```python
from build123d import *

# Parameters (mm, degrees)
F3_R     = 1.905
F7_W     = 78.89875
F7_H     = 0.5301288674
F8_DEPTH = 171.451


with BuildPart() as f1:
    # F0 (on Top) → F1 (revolve)
    with BuildSketch(Plane.XY):
        Polygon((-46.0375, 0), (-160.3375, 0), (-160.3375, -6.35), (-109.5375, -6.35), (-109.5375, -4.7625), (-84.1375, -4.7625), (-84.1375, -1.905), (84.1375, -1.905), (84.1375, -2.38125), (109.5375, -2.38125), (109.5375, -6.35), (134.9375, -6.35), (134.9375, -3.175), (160.3375, -3.175), (160.3375, 0), align=None)
    revolve(axis=Axis((40.7620462889, 0, 0), (1, 0, 0)))

    # F4: sweep along a path in F0
    with BuildLine(Plane.XY) as f4_path:
        Line((171.45, 73.81875), (45.1552021657, 73.81875))
        ThreePointArc((45.1552021657, 73.81875), (42.9987538677, 73.4413734385), (41.0986183394, 72.3540982639))
        Line((41.0986183394, 72.3540982639), (-46.0375, 0))
    # F3 (on plane+point) → F4 (sweep)
    with BuildSketch(Plane.YZ.offset(171.45)):
        with Locations((73.81875, 0)):
            Circle(F3_R)
    sweep(path=f4_path.line)

    # F5 (on Top) → F6 (revolve)
    with BuildSketch(Plane.XY):
        Polygon((95.25, 73.81875), (171.45, 73.81875), (171.45, 76.99375), (146.05, 76.99375), (146.05, 80.16875), (120.65, 80.16875), (120.65, 78.58125), (95.25, 78.58125), align=None)
    revolve(axis=Axis((128.362800926, 73.81875, 0), (1, 0, 0)))

    # F7 (on Right) → F8 (cut, through all)
    with BuildSketch(Plane.YZ):
        with Locations((36.909375, 6.0849355663)):
            Rectangle(F7_W, F7_H)
        with Locations((36.909375, -6.0849355663)):
            Rectangle(F7_W, F7_H)
    extrude(amount=F8_DEPTH, mode=Mode.SUBTRACT)


solid = f1.part
```
For this review, take the finished solid that the model builds, in its own axes (mm). A direction names the side the tool comes from. Round coordinates to 2 decimals unless told otherwise and drop trailing zeros. Write each loop counter-clockwise with the first axis right and the second up, starting at its lowest first coordinate (ties: lowest second). Pieces come first, ordered by that corner, then holes. Notation, with made-up numbers: (31.25, -27) - (52.25, -27) arc R34 cw to (52.25, 12) - close; hole circle Ø6 at (-25, -8.75). An arc over 180 degrees is marked (long way). Put each result on its own line as item: value.
Q1. We need section B-B (x = -81). Give the boundary of the cut face in (y, z) (3 decimals), and give its area (3 significant figures).
Solved:
outline: circle Ø3.81 at (0, 0)
area: 11.4 mm2
Q2. Machinability: for faces 5 (the face through (147.82, 0.69, 3.1)), 6 (the face through (-160.338, 0, 0)), 7 (the face through (-96.66, 3.78, 2.9)), 8 (the face through (160.338, 0, 0)), which of the approach directions +Z, -Z, +X, -X, +Y, -Y give a long, thin tool a straight path to every point of the face, cutting with its end or side? Answer none if there is none.
Solved:
face 5: +X
face 6: +Z, -Z, -X, +Y, -Y
face 7: none
face 8: +Z, -Z, +X, -Y
Q3. Wall thickness on probe 1 along Y at (x, z) = (129.5, 5.75); probe 2 along X at (y, z) = (1, -1.5); probe 3 along Y at (x, z) = (115.5, -2.75): over which ranges is each line inside the solid? List them lowest first.
Solved:
probe 1: y = -2.69 to 2.69, 71.12 to 76.51
probe 2: x = -160.34 to 160.34
probe 3: y = -5.72 to 5.72, 69.93 to 77.71
Q4. Insertion check: pin 1 Ø3 at (x, z) = (-98.5, -4) entering from +Y; pin 2 Ø3 at (y, z) = (75.5, -2) entering from -X; pin 3 Ø4 at (x, y) = (122.5, -0.5) entering from -Z. Each pin has a flat end and moves straight along its axis. Give the tip position at first contact, or say it passes through.
Solved:
pin 1: stops at y = 4.05
pin 2: stops at x = 41.18
pin 3: stops at z = -5.82
Q5. We need section A-A (x = 131). Give the boundary of the cut face in (y, z), and give its area (3 significant figures).
Solved:
outline: (-2.54, -5.82) - (2.54, -5.82) arc R6.35 ccw to (2.54, 5.82) - (-2.54, 5.82) arc R6.35 ccw to start; (71.28, -5.82) - (76.36, -5.82) arc R6.35 ccw to (76.36, 5.82) - (71.28, 5.82) arc R6.35 ccw to start
area: 246 mm2
Q6. Mouldability with a two-part tool opening along Y and no side actions: class faces 1 (the face through (133.172, 80.168, -0.103)), 2 (the face through (109.538, 0, -3)), 3 (the face through (171.45, 74, 0)), 4 (the face through (122.42, -6.35, 0.1)) as released by +Y, released by -Y, zero draft, split by the parting line, or undercut.
Solved:
face 1: released by +Y
face 2: undercut
face 3: zero draft
face 4: released by -Y
